Here's how the part is built. I have some questions about the finished solid (model axes, mm). Face numbers are marked on the shaded views. A direction names the side the tool comes from. Coordinates: 2 decimals unless noted, no trailing zeros. Loops run counter-clockwise (first coordinate to the right, second up) from the corner with the lowest first, then second, coordinate; pieces in that order, holes last. Notation, with made-up numbers: M 5.25,71.25 L 15.25,71.25 A9 ccw 15.25,86.25 Z; hole C 24,18.25 d2. An arc over 180 degrees is marked long. Use one line per item in the form item = value. Start each with the question number.
(1) Will these pins go through, and if not, where does the flat tip stop? P1, Ø6, axis at y = 45, z = 10, coming from the +X side; P2, Ø3.5, axis at y = 68.8, z = 13.6, coming from the -X side; P3, Ø4, axis at x = 30, y = 9, coming from the +Z side; P4, Ø5, axis at x = 48.5, z = 7, coming from the +Y side.
(2) Imagine slicing it at B-B, the plane x = 68. Please give me the cut outline in (y, z).
(3) Imagine slicing it at A-A, the plane z = 22.75. Please give me the cut outline in (x, y), and give its area (3 significant figures).
(4) On a 3-axis mill with a long thin cutter (end or side, diameter ignored), from which of +Z, -Z, +X, -X, +Y, -Y can I reach the whole of each face in a straight line? I mean the marked faces 1, 2, 3 and 4. Say none if no direction works.
(5) Please list where these lines run through material, in increasing order: L1, parallel to X at y = 25.8, z = 13.6; L2, parallel to X at y = 2.05, z = 13.6; L3, parallel to Y at x = 25.8, z = 13.6.
(6) Imagine slicing it at C-C, the plane x = 14. Please give me the cut outline in (y, z), and give its area (3 significant figures).
(7) Thinking about a two-plate mould opening in X: for the marked faces 5, 6 and 7, which applies, +X half, -X half, draft (parallel to the pull), parting line (faces both ways), or undercut?
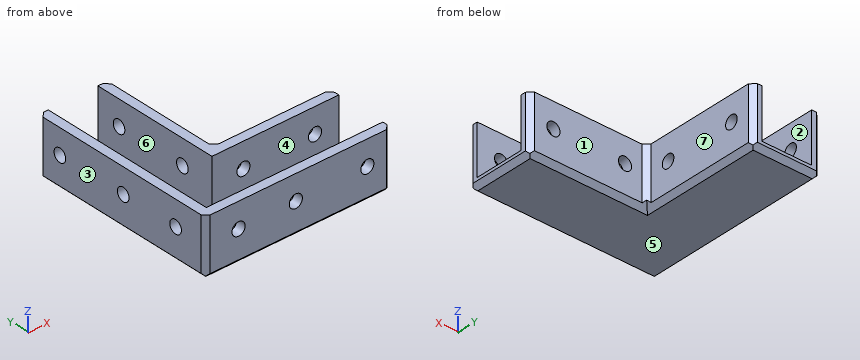
```python
from build123d import *

# Parameters (mm, degrees)
ESQUISSE2_W             = 28.8
ESQUISSE2_H             = 50
ESQUISSE2_W_2           = 78
ESQUISSE2_H_2           = 28.8
BOSS_EXTRU_2_DEPTH      = 24
ENL_V_MAT_EXTRU_1_DEPTH = 20.8
ESQUISSE4_R             = 2.75
ENL_V_MAT_EXTRU_2_DEPTH = 31.389271111
ESQUISSE5_R             = 2.75
ENL_V_MAT_EXTRU_3_DEPTH = 31.389271111
ESQUISSE6_R             = 2.75
ENL_V_MAT_EXTRU_4_DEPTH = 31.389271111
ESQUISSE7_R             = 2.75
ENL_V_MAT_EXTRU_5_DEPTH = 31.389271111
CHANFREIN1_SIZE         = 2
CHANFREIN2_SIZE         = 2


with BuildPart() as part:
    # Esquisse2 → Boss.-Extru.2 (new body)
    with BuildSketch(Plane.XY):
        with Locations((14.4, 53.8)):
            Rectangle(ESQUISSE2_W, ESQUISSE2_H)
        with Locations((39, 14.4)):
            Rectangle(ESQUISSE2_W_2, ESQUISSE2_H_2)
    extrude(amount=BOSS_EXTRU_2_DEPTH)

    # Esquisse3 → Enlèv. mat.-Extru.1 (cut)
    with BuildSketch(Plane.XY.offset(24)):
        Polygon((4, 78.8), (4, 4), (78, 4), (78, 24.8), (24.8, 24.8), (24.8, 78.8), align=None)
    extrude(amount=-ENL_V_MAT_EXTRU_1_DEPTH, mode=Mode.SUBTRACT)

    # Esquisse4 → Enlèv. mat.-Extru.2 (cut)
    with BuildSketch(Plane(origin=(0, 28.8, 0), x_dir=(1, 0, 0), z_dir=(0, 1, 0))):
        with Locations(Location((68, -13.6, 0), (0, 0, 270))):
            Circle(ESQUISSE4_R)
        with Locations(Location((38, -13.6, 0), (0, 0, 270))):
            Circle(ESQUISSE4_R)
    extrude(amount=-ENL_V_MAT_EXTRU_2_DEPTH, mode=Mode.SUBTRACT)

    # Esquisse5 → Enlèv. mat.-Extru.3 (cut)
    with BuildSketch(Plane(origin=(28.8, 0, 0), x_dir=(0, 0, -1), z_dir=(1, 0, 0))):
        with Locations(Location((-13.6, 38.8, 0), (0, 0, 270))):
            Circle(ESQUISSE5_R)
        with Locations(Location((-13.6, 68.8, 0), (0, 0, 270))):
            Circle(ESQUISSE5_R)
    extrude(amount=-ENL_V_MAT_EXTRU_3_DEPTH, mode=Mode.SUBTRACT)

    # Esquisse6 → Enlèv. mat.-Extru.4 (cut)
    with BuildSketch(Plane.ZY):
        with Locations((13.6, 14)):
            Circle(ESQUISSE6_R)
    extrude(amount=-ENL_V_MAT_EXTRU_4_DEPTH, mode=Mode.SUBTRACT)

    # Esquisse7 → Enlèv. mat.-Extru.5 (cut)
    with BuildSketch(Plane.XZ):
        with Locations(Location((14, 13.6, 0), (0, 0, 270))):
            Circle(ESQUISSE7_R)
    extrude(amount=-ENL_V_MAT_EXTRU_5_DEPTH, mode=Mode.SUBTRACT)

    # Chanfrein1
    chanfrein1_edges = [part.edges().sort_by_distance(p)[0] for p in [
        (28.8, 53.8, 0),
        (53.4, 28.8, 0),
        (39, 0, 0),
        (0, 39.4, 0),
    ]]
    chamfer(chanfrein1_edges, length=CHANFREIN1_SIZE)

    # Chanfrein2
    # the kernel refuses this chamfer: 2 mm, written as the material it adds along each edge
    with BuildSketch(Plane(origin=(28.8, 28.8, -3.143365976), x_dir=(-0.027495876610585647, 0.9996219169112968, 0), z_dir=(0, 0, 1))) as chanfrein2_piece_1_section:
        Polygon((CHANFREIN2_SIZE * 0.999621916911, -CHANFREIN2_SIZE * 0.0274958766106), (-CHANFREIN2_SIZE * 0.0274958766106, -CHANFREIN2_SIZE * 0.999621916911), (0, 0), align=None)
    chanfrein2_piece_1 = extrude(amount=27.143365976, mode=Mode.PRIVATE)
    chanfrein2_piece_1 = split(chanfrein2_piece_1, bisect_by=Plane(origin=(29.819330427, 29.005558504, 3.019330427), z_dir=(0.7071067811865476, 0, -0.7071067811865476)), keep=Keep.TOP, mode=Mode.PRIVATE)
    chanfrein2_piece_1 = split(chanfrein2_piece_1, bisect_by=Plane(origin=(30.090587735, 29.276815812, 2.476815812), z_dir=(0, -0.7071067811865476, 0.7071067811865476)), keep=Keep.TOP, mode=Mode.PRIVATE)
    add(chanfrein2_piece_1)
    with BuildSketch(Plane(origin=(28.8, 28.8, -3.143365976), x_dir=(-0.027495876610585647, 0.9996219169112968, 0), z_dir=(0, 0, 1))) as chanfrein2_piece_2_section:
        Polygon((CHANFREIN2_SIZE * 0.999621916911, -CHANFREIN2_SIZE * 0.0274958766106), (-CHANFREIN2_SIZE * 0.0274958766106, -CHANFREIN2_SIZE * 0.999621916911), (0, 0), align=None)
    chanfrein2_piece_2 = extrude(amount=27.143365976, mode=Mode.PRIVATE)
    chanfrein2_piece_2 = split(chanfrein2_piece_2, bisect_by=Plane(origin=(29.276815812, 30.090587735, 2.476815812), z_dir=(-0.7071067811865476, 0, 0.7071067811865476)), keep=Keep.TOP, mode=Mode.PRIVATE)
    chanfrein2_piece_2 = split(chanfrein2_piece_2, bisect_by=Plane(origin=(29.005558504, 29.819330427, 3.019330427), z_dir=(0, 0.7071067811865476, -0.7071067811865476)), keep=Keep.TOP, mode=Mode.PRIVATE)
    add(chanfrein2_piece_2)
    with BuildSketch(Plane(origin=(28.8, 28.8, -3.143365976), x_dir=(-0.027495876610585647, 0.9996219169112968, 0), z_dir=(0, 0, 1))) as chanfrein2_piece_3_section:
        Polygon((CHANFREIN2_SIZE * 0.999621916911, -CHANFREIN2_SIZE * 0.0274958766106), (-CHANFREIN2_SIZE * 0.0274958766106, -CHANFREIN2_SIZE * 0.999621916911), (0, 0), align=None)
    chanfrein2_piece_3 = extrude(amount=27.143365976, mode=Mode.PRIVATE)
    chanfrein2_piece_3 = split(chanfrein2_piece_3, bisect_by=Plane(origin=(34.880092378, 29.455254944, 8.080092378), z_dir=(-0.7071067811865476, 0, 0.7071067811865476)), keep=Keep.TOP, mode=Mode.PRIVATE)
    chanfrein2_piece_3 = split(chanfrein2_piece_3, bisect_by=Plane(origin=(29.455254944, 34.880092378, 8.080092378), z_dir=(0, -0.7071067811865476, 0.7071067811865476)), keep=Keep.TOP, mode=Mode.PRIVATE)
    add(chanfrein2_piece_3)
    # the kernel refuses this chamfer: 2 mm, written as the material it takes off along each edge
    with BuildSketch(Plane(origin=(0, 0, -3.143365976), x_dir=(-0.027495876610586372, 0.9996219169112968, 0), z_dir=(0, 0, 1)), Plane(origin=(28.8, 78.8, -3.143365976), x_dir=(0.02749587661058555, -0.9996219169112968, 0), z_dir=(0, 0, 1)), Plane(origin=(78, 28.8, -3.143365976), x_dir=(0.0274958766105891, -0.9996219169112968, 0), z_dir=(0, 0, 1))) as chanfrein2_2_piece_1:
        Polygon((CHANFREIN2_SIZE * 0.999621916911, -CHANFREIN2_SIZE * 0.0274958766106), (-CHANFREIN2_SIZE * 0.0274958766106, -CHANFREIN2_SIZE * 0.999621916911), (0, 0), align=None)
    extrude(amount=32.286731952, mode=Mode.SUBTRACT)
    with BuildSketch(Plane(origin=(0, 78.8, -3.143365976), x_dir=(-0.027495876610586292, -0.9996219169112968, 0), z_dir=(0, 0, 1)), Plane(origin=(78, 0, -3.143365976), x_dir=(0.02749587661058908, 0.9996219169112968, 0), z_dir=(0, 0, 1))) as chanfrein2_2_piece_2:
        Polygon((CHANFREIN2_SIZE * 0.999621916911, CHANFREIN2_SIZE * 0.0274958766106), (-CHANFREIN2_SIZE * 0.0274958766106, CHANFREIN2_SIZE * 0.999621916911), (0, 0), align=None)
    extrude(amount=32.286731952, mode=Mode.SUBTRACT)
    with BuildSketch(Plane(origin=(31.943365976, 78.8, 0), x_dir=(0, -0.9996219169112968, -0.027495876610586292), z_dir=(-1, 0, 0))) as chanfrein2_2_piece_3:
        Polygon((CHANFREIN2_SIZE * 0.999621916911, CHANFREIN2_SIZE * 0.0274958766106), (-CHANFREIN2_SIZE * 0.0274958766106, CHANFREIN2_SIZE * 0.999621916911), (0, 0), align=None)
    extrude(amount=35.086731952, mode=Mode.SUBTRACT)
    with BuildSketch(Plane(origin=(78, -3.143365976, 0), x_dir=(0.02749587661058908, 0, 0.9996219169112968), z_dir=(0, 1, 0))) as chanfrein2_2_piece_4:
        Polygon((CHANFREIN2_SIZE * 0.999621916911, -CHANFREIN2_SIZE * 0.0274958766106), (-CHANFREIN2_SIZE * 0.0274958766106, -CHANFREIN2_SIZE * 0.999621916911), (0, 0), align=None)
    extrude(amount=35.086731952, mode=Mode.SUBTRACT)


solid = part.part
```
Answer:
q1.P1 = 28.8
q1.P2 = through
q1.P3 = 3.2
q1.P4 = 28.8
q2.outline = M 0,2 L 2,0 L 26.8,0 L 28.8,2 L 28.8,10.85 L 24.8,10.85 L 24.8,3.2 L 4,3.2 L 4,10.85 L 0,10.85 Z; M 0,16.35 L 4,16.35 L 4,24 L 0,24 Z; M 24.8,16.35 L 28.8,16.35 L 28.8,24 L 24.8,24 Z
q3.outline = M 0,2 L 2,0 L 76,0 L 78,2 L 78,4 L 4,4 L 4,78.8 L 2,78.8 L 0,76.8 Z; M 24.8,24.8 L 78,24.8 L 78,26.8 L 76,28.8 L 30.8,28.8 L 28.8,30.8 L 28.8,76.8 L 26.8,78.8 L 24.8,78.8 Z
q3.area = 1,020 mm²
q4.face_1 = +Z, -Z, +X, +Y
q4.face_2 = +Z, +Y
q4.face_3 = +Z, -Z, -X, +Y, -Y
q4.face_4 = +Z, +X
q5.L1 = 0 to 4, 24.8 to 35.25, 40.75 to 65.25, 70.75 to 78
q5.L2 = 0 to 11.25, 16.75 to 35.25, 40.75 to 65.25, 70.75 to 78
q5.L3 = 0 to 4, 24.8 to 36.05, 41.55 to 66.05, 71.55 to 78.8
q6.outline = M 0,2 L 2,0 L 76.8,0 L 78.8,2 L 78.8,3.2 L 4,3.2 L 4,10.85 L 0,10.85 Z; M 0,16.35 L 4,16.35 L 4,24 L 0,24 Z
q6.area = 309 mm²
q7.face_5 = draft
q7.face_6 = undercut
q7.face_7 = +X half
